For this review, take the finished solid that the model builds, in its own axes (mm). Face numbers are marked on the shaded views. A direction names the side the tool comes from. Give positions to 0.01 mm unless a question says otherwise; leave off trailing zeros. Order: outer loops, then holes, each group sorted by start corner. A loop starts at its lowest first (then second) coordinate and runs counter-clockwise, first axis right, second up. Notation, with made-up numbers: M 17,-30.5 L 62,-30.5 A31 ccw 62,-2.5 Z; hole C 85,-22.5 d7. An arc over 180 degrees is marked long. Answer as CSV lines item,"result". Start each with the question number.
1. We need section D-D, the plane x = 18.5. Give the boundary of the cut face in (y, z).
2. We need section B-B, the plane x = 57.15. Give the boundary of the cut face in (y, z), and give its area (3 significant figures).
3. Clearance check with flat-ended pins moving along their axes: P1, Ø19.5, axis at x = 22.5, z = 8.5, coming from the -Y side; P2, Ø2, axis at x = -14, z = 5.5, coming from the +Y side; P3, Ø6, axis at x = 3, y = 0, coming from the -Z side; P4, Ø3.5, axis at x = 57.15, y = 36.51, coming from the -Z side. State where each tip first meets the part, or that it passes through.
4. We need section A-A, the plane y = 0. Give the boundary of the cut face in (x, z).
5. Machinability: for the marked faces 1, 2, 3 and 4, which of the approach directions +Z, -Z, +X, -X, +Y, -Y give a long, thin tool a straight path to every point of the face, cutting with its end or side? Answer none if there is none.
6. Mouldability with a two-part tool opening along Z and no side actions: class the marked faces 5, 6 and 7 as pulls with the +Z half, pulls with the -Z half, needs draft (parallel to the pull), parting line crosses it, or undercut.
7. For line 1 along Y through (x, z) = (-57, -23); line 2 along Y through (x, z) = (-3, 4); line 3 along Z through (x, y) = (0, -33.5), list the stretches that pass through material, from the lowest coordinate up.
8. We need section C-C, the plane z = -1. Give the boundary of the cut face in (x, y).
from build123d import *

# Parameters (mm, degrees)
F0_R     = 12.7063531766
F1_DEPTH = 76.2
F2_R     = 2.794
F3_DEPTH = 9.6578284142


# Not quite as in the source:
# - ends of sketch curves that miss each other by under 0.0002 mm in the source are joined


with BuildPart() as f1:
    # F0 (on Right) → F1 (new body, symmetric)
    with BuildSketch(Plane.YZ):
        with BuildLine():
            Line((-41.2956478239, -26.3029134567), (-8.8944472236, -26.3029134567))
            Line((-8.8944472236, -26.3029134567), (-6.8614307154, -24.2698969485))
            Line((-6.8614307154, -24.2698969485), (6.8614307154, -24.2698969485))
            Line((6.8614307154, -24.2698969485), (8.8944472236, -26.3029134567))
            Line((8.8944472236, -26.3029134567), (41.2956478239, -26.3029134567))
            Line((41.2956478239, -26.3029134567), (41.2956478239, -16.6460850425))
            Line((41.2956478239, -16.6460850425), (30.2411205603, -16.6460850425))
            Line((30.2411205603, -16.6460850425), (30.2411205603, 22.7436098049))
            Line((30.2411205603, 22.7436098049), (29.9869934967, 22.9977368684))
            Line((29.9869934967, 22.9977368684), (16.8568834417, 22.9977368684))
            ThreePointArc((16.8568834417, 22.9977368684), (0, 29.3509134567), (-16.8568829775, 22.9977363401))
            Line((-16.8568829775, 22.9977363401), (-29.9869934967, 22.9977368684))
            Line((-29.9869934967, 22.9977368684), (-30.2411205603, 22.7436098049))
            Line((-30.2411205603, 22.7436098049), (-30.2411205603, -16.6460850425))
            Line((-30.2411205603, -16.6460850425), (-41.2956478239, -16.6460850425))
            Line((-41.2956478239, -16.6460850425), (-41.2956478239, -26.3029134567))
        make_face()
        with Locations((0, 3.8619689845)):
            Circle(F0_R, mode=Mode.SUBTRACT)
    extrude(amount=F1_DEPTH, both=True)

    # F2 (on face) → F3 (cut, through all)
    with BuildSketch(Plane.XY.offset(-16.6460850425)):
        with Locations((57.15, 36.5125)):
            Circle(F2_R)
        with Locations((-57.15, 36.5125)):
            Circle(F2_R)
        with Locations((-57.15, -36.5125)):
            Circle(F2_R)
        with Locations((57.15, -36.5125)):
            Circle(F2_R)
    extrude(amount=-F3_DEPTH, mode=Mode.SUBTRACT)


solid = f1.part
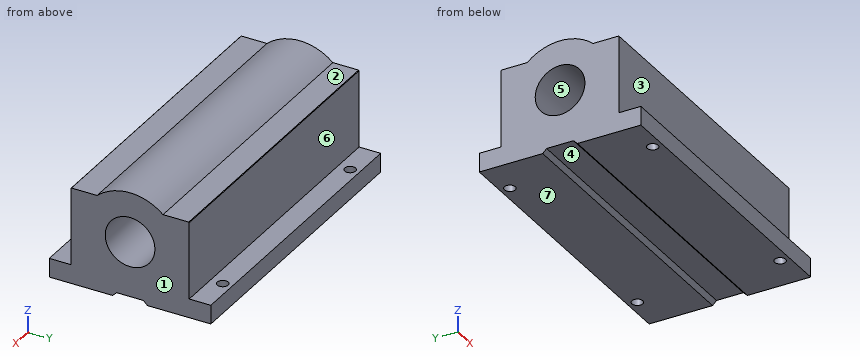
Result set:
1,outline,"M -41.3,-26.3 L -8.89,-26.3 L -6.86,-24.27 L 6.86,-24.27 L 8.89,-26.3 L 41.3,-26.3 L 41.3,-16.65 L 30.24,-16.65 L 30.24,22.74 L 29.99,23 L 16.86,23 A25.54 ccw -16.86,23 L -29.99,23 L -30.24,22.74 L -30.24,-16.65 L -41.3,-16.65 Z; hole C 0,3.86 d25.41"
2,outline,"M -41.3,-26.3 L -39.31,-26.3 L -39.31,-16.65 L -41.3,-16.65 Z; M -33.72,-26.3 L -8.89,-26.3 L -6.86,-24.27 L 6.86,-24.27 L 8.89,-26.3 L 33.72,-26.3 L 33.72,-16.65 L 30.24,-16.65 L 30.24,22.74 L 29.99,23 L 16.86,23 A25.54 ccw -16.86,23 L -29.99,23 L -30.24,22.74 L -30.24,-16.65 L -33.72,-16.65 Z; M 39.31,-26.3 L 41.3,-26.3 L 41.3,-16.65 L 39.31,-16.65 Z; hole C 0,3.86 d25.41"
2,area,"2,690 mm2"
3,P1,"y = -30.24"
3,P2,"y = 30.24"
3,P3,"z = -24.27"
3,P4,"through"
4,outline,"M -76.2,-24.27 L 76.2,-24.27 L 76.2,-8.84 L -76.2,-8.84 Z; M -76.2,16.57 L 76.2,16.57 L 76.2,29.35 L -76.2,29.35 Z"
5,face 1,"+Z, -Z, +X, +Y, -Y"
5,face 2,"+Z, +X, -X, +Y"
5,face 3,"+Z, +X, -X, -Y"
5,face 4,"-Z, +X, -X"
6,face 5,"undercut"
6,face 6,"needs draft"
6,face 7,"pulls with the -Z half"
7,line 1,"-41.3 to -39.3, -33.72 to 33.72, 39.3 to 41.3"
7,line 2,"-30.24 to -12.71, 12.71 to 30.24"
7,line 3,"-26.3 to -16.65"
8,outline,"M -76.2,-30.24 L 76.2,-30.24 L 76.2,-11.74 L -76.2,-11.74 Z; M -76.2,11.74 L 76.2,11.74 L 76.2,30.24 L -76.2,30.24 Z"
